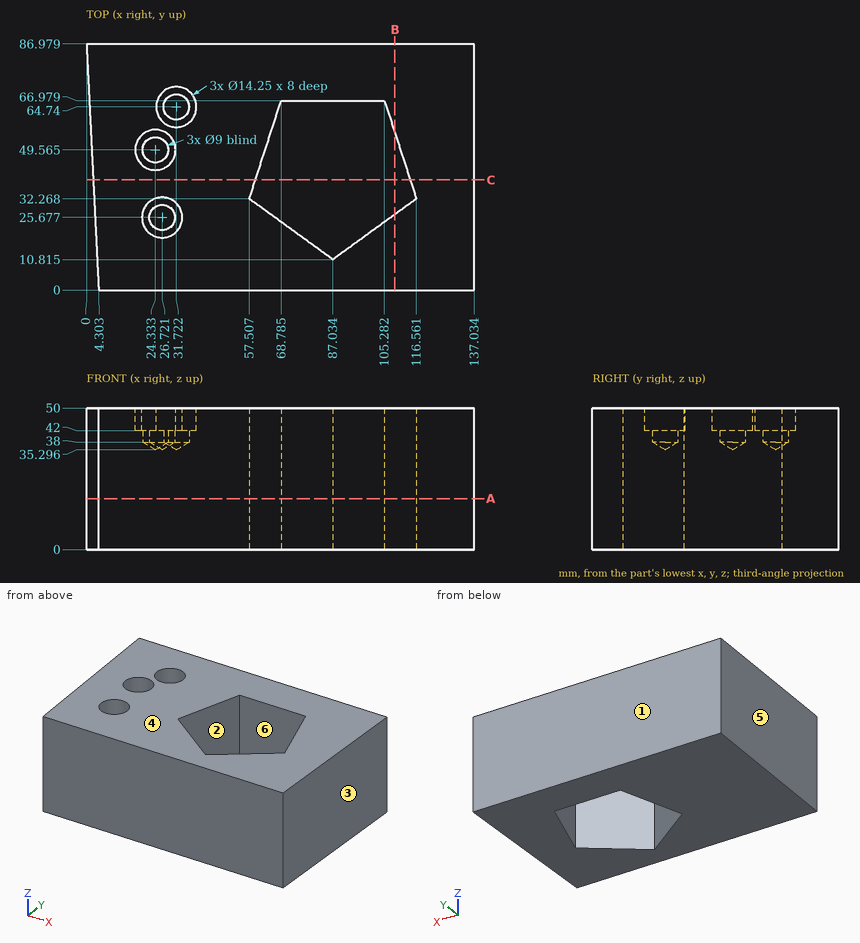
Could you check a few things on this drawing? It's one solid part, dimensions in mm from its lowest x, y, z. A direction names the side the tool comes from. Round coordinates to 2 decimals unless told otherwise and drop trailing zeros. Write each loop counter-clockwise with the first axis right and the second up, starting at its lowest first coordinate (ties: lowest second). Pieces come first, ordered by that corner, then holes.
Q1. Please list where these lines run through material, in increasing order: probe 1 along X at (y, z) = (23, 39) (1 decimal); probe 2 along X at (y, z) = (23.5, 37.5) (1 decimal); probe 3 along Y at (x, z) = (78, 8).
Q2. Will these pins go through, and if not, where does the flat tip stop? P1, Ø4.5, axis at x = 27, y = 52, coming from the +Z side; P2, Ø2, axis at y = 50.5, z = 25.5, coming from the -X side (1 decimal); P3, Ø12, axis at y = 23, z = 20, coming from the -X side.
Q3. Which directions (+Z, -Z, +X, -X, +Y, -Y) give clear straight access to the entire face, cutting with the end or side of a thin tool? Please do the marked faces 1 and 2.
Q4. If we section it at B-B on x = 109: Write out the boundary of the cut face in (y, z) (1 decimal), plus the area to 3 significant figures.
Q5. If we section it at A-A on z = 18: Write out the boundary of the cut face in (x, y) (1 decimal), plus the area to 3 significant figures.
Q6. If we section it at C-C on y = 39: Write out the boundary of the cut face in (x, z) (1 decimal), plus the area to 3 significant figures.
Q7. If we mould it in two halves opening along X, with no side actions, what happens to the marked faces 3, 4, 5 and 6? For each: +X half, -X half, draft (parallel to the pull), parting line (faces both ways), or undercut.
Answer below:
1. probe 1: x = 3.2 to 23.1, 30.3 to 70.3, 103.8 to 137
1. probe 2: x = 3.1 to 23.8, 29.7 to 69.6, 104.5 to 137
1. probe 3: y = 0 to 17.38, 66.98 to 86.98
2. P1: stops at z = 42
2. P2: stops at x = 1.8
2. P3: stops at x = 2.87
3. face 1: +Z, -Z, +X, -X, +Y
3. face 2: +Z, -Z
4. outline: (0, 0) - (26.8, 0) - (26.8, 50) - (0, 50) - close; (55.5, 0) - (87, 0) - (87, 50) - (55.5, 50) - close
4. area: 2,910 mm2
5. outline: (0, 87) - (4.3, 0) - (137, 0) - (137, 87) - close; hole (57.5, 32.3) - (87, 10.8) - (116.6, 32.3) - (105.3, 67) - (68.8, 67) - close
5. area: 9,440 mm2
6. outline: (2.4, 0) - (59.7, 0) - (59.7, 50) - (2.4, 50) - close; (114.4, 0) - (137, 0) - (137, 50) - (114.4, 50) - close
6. area: 4,000 mm2
7. face 3: +X half
7. face 4: draft
7. face 5: -X half
7. face 6: undercut
